Verification items for the finished model (mm, model axes). Face numbers are marked on the shaded views. A direction names the side the tool comes from. Round coordinates to 2 decimals unless told otherwise and drop trailing zeros. Write each loop counter-clockwise with the first axis right and the second up, starting at its lowest first coordinate (ties: lowest second). Pieces come first, ordered by that corner, then holes. Notation, with made-up numbers: (-18, -36) - (16, -36) arc R24 cw to (16, -21) - close; hole circle Ø8 at (32, -8). An arc over 180 degrees is marked (long way). Write each question's results on one line, items separated by ' | '.
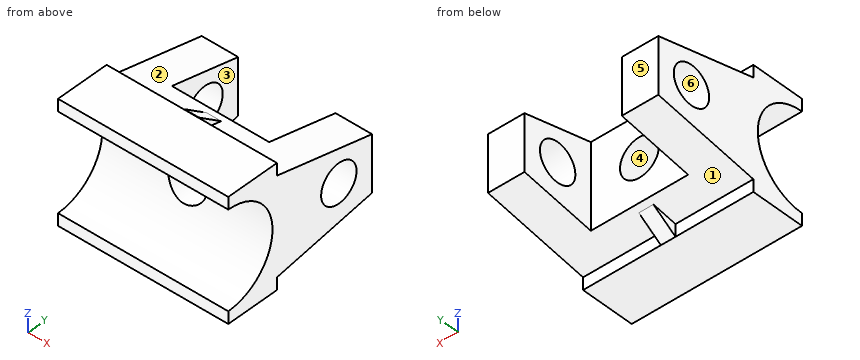
```python
from build123d import *

# Parameters (mm, degrees)
SKETCH1_W               = 140
SKETCH1_H               = 100
BOSS_EXTRUDE1_DEPTH     = 44
CUT_EXTRUDE2_DEPTH      = 1
CUT_EXTRUDE2_DEPTH_BACK = 141
BOSS_EXTRUDE2_DEPTH     = 140
SKETCH5_W               = 80
SKETCH5_H               = 60
CUT_EXTRUDE3_DEPTH      = 1
CUT_EXTRUDE3_DEPTH_BACK = 101
SKETCH6_R               = 16
CUT_EXTRUDE4_DEPTH      = 61
CUT_EXTRUDE4_DEPTH_BACK = 71
SKETCH7_R               = 16
CUT_EXTRUDE5_DEPTH      = 1.0000001
CUT_EXTRUDE5_DEPTH_BACK = 141.0000001
BOSS_EXTRUDE6_DEPTH     = 6
BOSS_EXTRUDE7_DEPTH     = 6


with BuildPart() as part:
    # Sketch1 → Boss-Extrude1 (new body)
    with BuildSketch(Plane(origin=(0, 0, 0), x_dir=(1, 0, 0), z_dir=(0, 1, 0))):
        with Locations((70, 50)):
            Rectangle(SKETCH1_W, SKETCH1_H)
    extrude(amount=BOSS_EXTRUDE1_DEPTH)

    # Sketch2 → Cut-Extrude2 (cut, two sides)
    with BuildSketch(Plane.ZY) as cut_extrude2_sk:
        with BuildLine():
            Line((-90, -210.359676582), (-90, 0))
            ThreePointArc((-90, 0), (-50, 40), (-10, 0))
            Line((-10, 0), (-10, -210.359676582))
            Line((-10, -210.359676582), (-10, -631.079029746))
            Line((-10, -631.079029746), (-90, -631.079029746))
            Line((-90, -631.079029746), (-90, -210.359676582))
        make_face()
    extrude(amount=CUT_EXTRUDE2_DEPTH, mode=Mode.SUBTRACT)
    extrude(cut_extrude2_sk.sketch, amount=-CUT_EXTRUDE2_DEPTH_BACK, mode=Mode.SUBTRACT)

    # Sketch3 → Boss-Extrude2 (add)
    with BuildSketch(Plane.ZY):
        Polygon((-90, 44), (-75.775374972, 130), (-29.52448448, 130), (-10, 44), align=None)
    extrude(amount=-BOSS_EXTRUDE2_DEPTH)

    # Sketch5 → Cut-Extrude3 (cut, two sides)
    with BuildSketch(Plane.XY) as cut_extrude3_sk:
        with Locations((70, 100)):
            Rectangle(SKETCH5_W, SKETCH5_H)
    extrude(amount=CUT_EXTRUDE3_DEPTH, mode=Mode.SUBTRACT)
    extrude(cut_extrude3_sk.sketch, amount=-CUT_EXTRUDE3_DEPTH_BACK, mode=Mode.SUBTRACT)

    # Sketch6 → Cut-Extrude4 (cut, two sides)
    with BuildSketch(Plane(origin=(0, 70, 0), x_dir=(1, 0, 0), z_dir=(0, 1, 0))) as cut_extrude4_sk:
        with Locations((70, 50)):
            Circle(SKETCH6_R)
    extrude(amount=CUT_EXTRUDE4_DEPTH, mode=Mode.SUBTRACT)
    extrude(cut_extrude4_sk.sketch, amount=-CUT_EXTRUDE4_DEPTH_BACK, mode=Mode.SUBTRACT)

    # Sketch7 → Cut-Extrude5 (cut, two sides)
    with BuildSketch(Plane.ZY) as cut_extrude5_sk:
        with Locations((-50, 100)):
            Circle(SKETCH7_R)
    extrude(amount=CUT_EXTRUDE5_DEPTH, mode=Mode.SUBTRACT)
    extrude(cut_extrude5_sk.sketch, amount=-CUT_EXTRUDE5_DEPTH_BACK, mode=Mode.SUBTRACT)

    # Sketch15 → Boss-Extrude6 (add, symmetric)
    with BuildSketch(Plane.ZY.offset(-70)):
        Polygon((-14.540577786, 64), (-10, 44), (0.380318398, 44), align=None)
    extrude(amount=BOSS_EXTRUDE6_DEPTH, both=True)

    # Sketch17 → Boss-Extrude7 (add, symmetric)
    with BuildSketch(Plane.ZY.offset(-70)):
        Polygon((-86.691947668, 64), (-100.019037355, 44), (-90, 44), align=None)
    extrude(amount=BOSS_EXTRUDE7_DEPTH, both=True)


solid = part.part
```
(1) Section check C-C (y = 100). Record the cut outline in (x, z).
Answer:
outline: (0, -80.74) - (30, -80.74) - (30, -66) - (0, -66) - close; (0, -34) - (30, -34) - (30, -22.71) - (0, -22.71) - close; (110, -80.74) - (140, -80.74) - (140, -66) - (110, -66) - close; (110, -34) - (140, -34) - (140, -22.71) - (110, -22.71) - close
(2) Go/stop test with flat-tipped pins: pin 1 Ø3 at (x, z) = (116, -4.5) entering from +Y; pin 2 Ø21 at (x, z) = (78.5, -60) entering from +Y; pin 3 Ø3 at (x, y) = (101.5, 44.5) entering from -Z. Record where each tip stops, or that it passes through.
Answer:
pin 1: y = 44 | pin 2: y = 70 | pin 3: z = -100
(3) Set-up check for the marked faces 1, 2 and 3: record each of +Z, -Z, +X, -X, +Y, -Y from which the full face is reachable in a straight line by a thin tool's end or side.
Answer:
face 1: -Z, +Y | face 2: +Z, +Y | face 3: +Z, -Z, +Y
(4) Section check A-A (z = -50). Record the cut outline in (x, y), plus the area to 3 significant figures.
Answer:
outline: (0, 40) - (54, 40) - (54, 70) - (30, 70) - (30, 84) - (0, 84) - close; (0, 116) - (30, 116) - (30, 130) - (0, 130) - close; (86, 40) - (140, 40) - (140, 84) - (110, 84) - (110, 70) - (86, 70) - close; (110, 116) - (140, 116) - (140, 130) - (110, 130) - close | area: 4,920 mm2
(5) Thickness scan on L1, parallel to Y at x = 122.5, z = -50; L2, parallel to X at y = 80, z = -45; L3, parallel to X at y = 50, z = -50. Record the ranges inside material, lowest first.
Answer:
L1: 40 to 84, 116 to 130 | L2: 0 to 30, 110 to 140 | L3: 0 to 54, 86 to 140
(6) Mould release check, pull along Y, two halves, no side actions. Record for the marked faces 4, 5 and 6: released by +Y, released by -Y, zero draft, split by the parting line, or undercut.
Answer:
face 4: zero draft | face 5: released by +Y | face 6: undercut
(7) Section check D-D (y = 18). Record the cut outline in (x, z).
Answer:
outline: (0, -100) - (140, -100) - (140, -85.72) - (0, -85.72) - close; (0, -14.28) - (140, -14.28) - (140, 0) - (0, 0) - close
